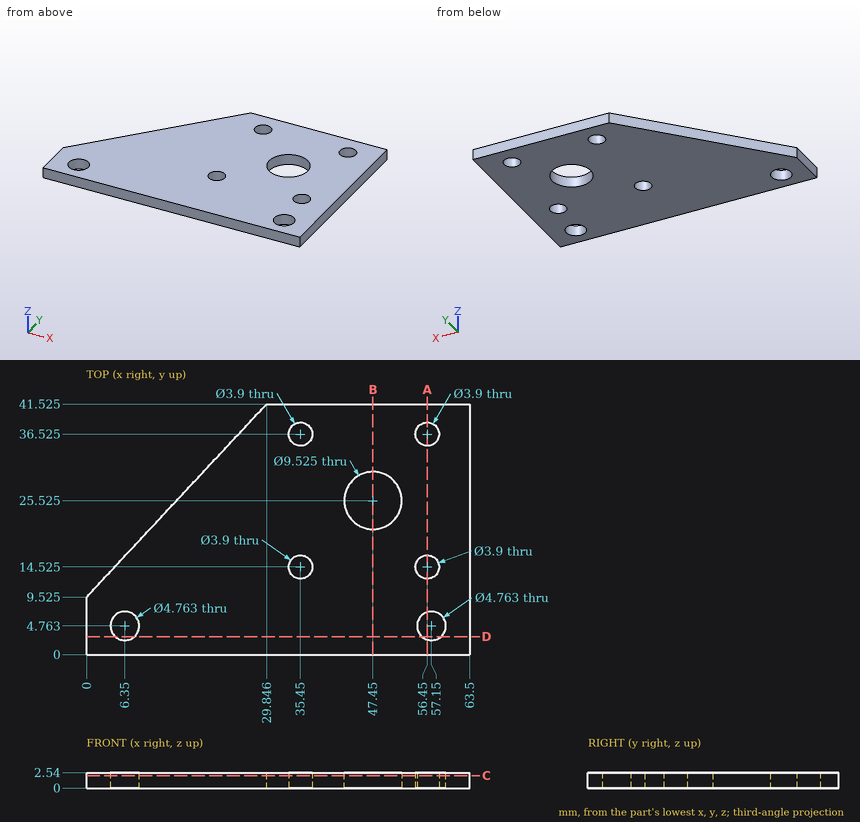
Print and shaded views of the part. All mm, measured from the part's lowest x, y and z. Coordinates: 2 decimals unless noted, no trailing zeros. Loops run counter-clockwise (first coordinate to the right, second up) from the corner with the lowest first, then second, coordinate; pieces in that order, holes last. Notation, with made-up numbers: M -26,59.5 L 17,59.5 A30 ccw 17,90.5 Z; hole C 3,11 d5. An arc over 180 degrees is marked long. Use a Markdown table: item, result. Add a question column.
Q1. Cut at D-D (y = 3). Write the cut outline in (x, z).
Q2. Cut at C-C (z = 2.05). Give the number of separate pieces and of enclosed holes in the cut face, and give its area (3 significant figures).
Q3. Cut at A-A (x = 56.45). Write the cut outline in (y, z) (1 decimal).
Q4. Cut at B-B (x = 47.45). Write the cut outline in (y, z) (1 decimal).
Q5. Pin check, flat tip, straight feed: P1, Ø2.5, axis at x = 56.45, y = 14.525, coming from the -Z side. Stop position of the tip, or through.
Q6. Probe L1, parallel to Y at x = 35.45, z = 0.7 (1 decimal); L2, parallel to X at y = 5, z = 1.4; L3, parallel to X at y = 16, z = 1.1 (1 decimal). List the from-to ranges inside material, lowest first.
Worked out:
| question | item | result |
|---|---|---|
| 1 | outline | M 0,0 L 4.75,0 L 4.75,2.54 L 0,2.54 Z; M 7.95,0 L 55.55,0 L 55.55,2.54 L 7.95,2.54 Z; M 58.75,0 L 63.5,0 L 63.5,2.54 L 58.75,2.54 Z |
| 2 | separate pieces | 1 |
| 2 | enclosed holes | 7 |
| 2 | area | 2,000 mm2 |
| 3 | outline | M 0,0 L 2.5,0 L 2.5,2.5 L 0,2.5 Z; M 7,0 L 12.6,0 L 12.6,2.5 L 7,2.5 Z; M 16.5,0 L 34.6,0 L 34.6,2.5 L 16.5,2.5 Z; M 38.5,0 L 41.5,0 L 41.5,2.5 L 38.5,2.5 Z |
| 4 | outline | M 0,0 L 20.8,0 L 20.8,2.5 L 0,2.5 Z; M 30.3,0 L 41.5,0 L 41.5,2.5 L 30.3,2.5 Z |
| 5 | P1 | passes through |
| 6 | L1 | y = 0 to 12.6, 16.5 to 34.6, 38.5 to 41.5 |
| 6 | L2 | x = 0 to 3.98, 8.72 to 54.78, 59.52 to 63.5 |
| 6 | L3 | x = 6 to 34.2, 36.7 to 55.2, 57.7 to 63.5 |
